Could you check a few things on this model? Use its own coordinates, in mm. A direction names the side the tool comes from. Coordinates: 2 decimals unless noted, no trailing zeros. Write each loop counter-clockwise with the first axis right and the second up, starting at its lowest first coordinate (ties: lowest second). Pieces come first, ordered by that corner, then holes. Notation, with made-up numbers: M 26,44 L 65,44 A15 cw 65,57 Z; hole C 35,-6.75 d10. An arc over 180 degrees is marked long. Answer as CSV lines item,"result". Start each with the question number.
Item 1: Suppose I cut it at C-C, the plane z = -13. Write out the boundary of the cut face in (x, y) (3 decimals), and give its area (3 significant figures).
Item 2: If I drill on line 1 along Z through (x, y) = (16.5, 3.75) (3 decimals); line 2 along X through (y, z) = (2.4, 11.5) (3 decimals); line 3 along X through (y, z) = (0.85, 1), over which ranges is the centre line in solid material (lowest first)? Write a range as [from, to].
Item 3: Suppose I cut it at B-B, the plane y = 4.75. State how many separate pieces and enclosed holes the cut face has, and give its area (3 significant figures).
Item 4: Suppose I cut it at D-D, the plane x = 1. Write out the boundary of the cut face in (y, z), and give its area (3 significant figures).
Item 5: I'm going to push flat-ended pins straight in: P1, Ø2, axis at y = 5, z = -14.5, coming from the +X side (3 decimals); P2, Ø0.9, axis at x = -0.5, y = 2.5, coming from the -Z side; P3, Ø3, axis at x = 18.5, y = 4, coming from the -Z side (3 decimals); P4, Ø5, axis at x = -8, z = -15, coming from the +Y side. Where does each tip first touch, or does it pass through?
Item 6: Suppose I cut it at A-A, the plane x = 18. Write out the boundary of the cut face in (y, z) (3 decimals), and give its area (3 significant figures).
Item 7: We'd pull the mould along X, two halves only. Please class faces 6 (the flat face through (21.717, 3, 3)), 7 (the cylindrical face through (12.78, 2.96, -31.5)), 8 (the flat face through (0.584, 2.962, 5.749)): +X half, -X half, draft (parallel to the pull), parting line (faces both ways), or undercut.
Item 8: On a 3-axis mill with a long thin cutter (end or side, diameter ignored), from which of +Z, -Z, +X, -X, +Y, -Y can I reach the whole of each face in a straight line? I mean faces 1 (the flat face through (-9.525, 3, -6)), 2 (the flat face through (-12, 3, 9.525)), 3 (the flat face through (19, 3, -3.175)), 4 (the flat face through (1.42, 2.96, -11.49)), 5 (the flat face through (15.875, 3, -30)). Say none if no direction works.
```python
from build123d import *

# Parameters (mm, degrees)
BOSS_EXTRUDE1_DEPTH = 5.842
CUT_EXTRUDE1_DEPTH  = 39.907834083
FILLET1_R           = 3.175
FILLET2_R           = 1.5875
FILLET3_R           = 3.175
SKETCH3_W           = 25.4
SKETCH3_H           = 3.175
CUT_EXTRUDE2_DEPTH  = 39.907834083


with BuildPart() as part:
    # Sketch1 → Boss-Extrude1 (new body)
    with BuildSketch(Plane(origin=(0, 0, 0), x_dir=(1, 0, 0), z_dir=(0, 1, 0))):
        Polygon((15.875, -15.875), (-9.525, -15.875), (-9.525, -9.525), (-15.367, -9.525), (-15.367, 3.175), (-9.525, 3.175), (-9.525, 9.525), (12.7, 31.75), (15.875, 31.75), (15.875, 28.575), (21.717, 28.575), (21.717, 15.875), (15.875, 15.875), (15.875, 3.175), (21.717, 3.175), (21.717, -9.525), (15.875, -9.525), align=None)
    extrude(amount=BOSS_EXTRUDE1_DEPTH)

    # Sketch2 → Cut-Extrude1 (cut, through all)
    with BuildSketch(Plane(origin=(0, 5.842, 0), x_dir=(1, 0, 0), z_dir=(0, 1, 0))):
        Polygon((-3.175, 6.894743879), (9.525, 19.594743879), (9.525, -9.525), align=None)
        Polygon((-3.175, -0.889537058), (3.504177225, -9.525), (-3.175, -9.525), align=None)
    extrude(amount=-CUT_EXTRUDE1_DEPTH, mode=Mode.SUBTRACT)

    # Fillet1
    fillet1_edges = [part.edges().sort_by_distance(p)[0] for p in [
        (12.7, 2.921, -31.75),
    ]]
    fillet(fillet1_edges, radius=FILLET1_R)

    # Fillet2
    fillet2_edges = [part.edges().sort_by_distance(p)[0] for p in [
        (-3.175, 2.921, 9.525),
        (-3.175, 2.921, 0.889537058),
        (3.504177225, 2.921, 9.525),
    ]]
    fillet(fillet2_edges, radius=FILLET2_R)

    # Fillet3
    fillet3_edges = [part.edges().sort_by_distance(p)[0] for p in [
        (9.525, 2.921, 9.525),
        (-3.175, 2.921, -6.894743879),
        (9.525, 2.921, -19.594743879),
    ]]
    fillet(fillet3_edges, radius=FILLET3_R)

    # Sketch3 → Cut-Extrude2 (cut, through all)
    with BuildSketch(Plane(origin=(0, 5.842, 0), x_dir=(1, 0, 0), z_dir=(0, 1, 0))):
        with Locations((3.175, -14.2875)):
            Rectangle(SKETCH3_W, SKETCH3_H)
    extrude(amount=-CUT_EXTRUDE2_DEPTH, mode=Mode.SUBTRACT)


solid = part.part
```
Ans:
1,outline,"M -6.05,0 L 2.93,0 L 2.93,5.842 L -6.05,5.842 Z; M 9.339,0 L 15.875,0 L 15.875,5.842 L 9.339,5.842 Z"
1,area,"90.6 mm^2"
2,line 1,"z = [-28.575, -15.875], [-3.175, 9.525]"
2,line 2,"x = [-9.525, 15.875]"
2,line 3,"x = [-15.37, 2.93], [9.43, 21.72]"
3,separate pieces,"1"
3,enclosed holes,"2"
3,area,"929 mm^2"
4,outline,"M 0,-20.05 L 5.84,-20.05 L 5.84,-11.07 L 0,-11.07 Z; M 0,-1.5 L 5.84,-1.5 L 5.84,6.29 L 0,6.29 Z; M 0,9.35 L 5.84,9.35 L 5.84,12.7 L 0,12.7 Z"
4,area,"118 mm^2"
5,P1,"stops at x = 15.875"
5,P2,"stops at z = -19"
5,P3,"stops at z = -28.575"
5,P4,"passes through"
6,outline,"M 0,-28.575 L 5.842,-28.575 L 5.842,-15.875 L 0,-15.875 Z; M 0,-3.175 L 5.842,-3.175 L 5.842,9.525 L 0,9.525 Z"
6,area,"148 mm^2"
7,face 6,"+X half"
7,face 7,"-X half"
7,face 8,"undercut"
8,face 1,"-Z, -X, +Y, -Y"
8,face 2,"+Z, -X, +Y, -Y"
8,face 3,"+X, +Y, -Y"
8,face 4,"+Y, -Y"
8,face 5,"-Z, +X, +Y, -Y"
